from build123d import *

# Parameters (mm, degrees)
PAD003_DEPTH = 30
SKETCH005_R  = 6
POCKET_DEPTH = 30.001
SKETCH006_R  = 4.232151
PAD004_DEPTH = 20


with BuildPart() as part:
    # Sketch004 → Pad003 (new body)
    with BuildSketch(Plane.XY):
        Polygon((-12, 0), (-15, 0), (-15, 50), (15, 50), (15, 0), (12, 0), (12, 47), (-12, 47), align=None)
    extrude(amount=PAD003_DEPTH)

    # Sketch005 (on DatumPlane) → Pocket (cut, through all)
    with BuildSketch(Plane.YZ.offset(15)):
        with Locations((10, 15.016033)):
            Circle(SKETCH005_R)
    extrude(amount=-POCKET_DEPTH, mode=Mode.SUBTRACT)

    # Sketch006 (on DatumPlane) → Pad004 (join)
    with BuildSketch(Plane(origin=(0, 50, 0), x_dir=(-1, 0, 0), z_dir=(0, 1, 0))):
        with Locations((0, 15)):
            Circle(SKETCH006_R)
    extrude(amount=PAD004_DEPTH)


with BuildPart() as part_1:
    # Body009 placement: moved
    add(part.part.moved(Location((10, -300, 0))))


solid = part_1.part
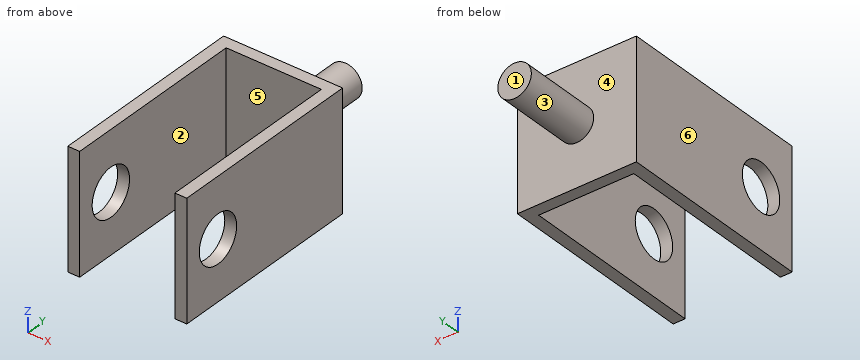
Source: CAD feature listing. Evaluate the final solid. Frame: model axes, mm. Face numbers are marked on the shaded views. A direction names the side the tool comes from. Coordinates: 2 decimals unless noted, no trailing zeros. Loops run counter-clockwise (first coordinate to the right, second up) from the corner with the lowest first, then second, coordinate; pieces in that order, holes last. Notation, with made-up numbers: (7, -33.5) - (11, -33.5) arc R22 cw to (11, -18.5) - close; hole circle Ø2 at (47.5, -13). An arc over 180 degrees is marked (long way). One line per question, with ' | ' between items.
1) Section C-C, the plane z = 22. Return loops of the section in (x, y).
Report:
outline: (-5, -300) - (-2, -300) - (-2, -253) - (22, -253) - (22, -300) - (25, -300) - (25, -250) - (-5, -250) - close
2) First-contact query: P1, Ø3, axis at x = 15.5, z = 4, coming from the -Y side; P2, Ø2, axis at y = -245.5, z = 21.5, coming from the +X side; P3, Ø3, axis at x = 14, z = 21.5, coming from the +Y side; P4, Ø15.5, axis at y = -290, z = 15.02, coming from the -X side. Flat tips, straight axial feed; report the tip coordinate or a pass-through.
Report:
P1: stops at y = -253 | P2: passes through | P3: stops at y = -250 | P4: stops at x = -5
3) Section A-A, the plane y = -280. Return loops of the section in (x, z), then the cut area to 3 significant figures.
Report:
outline: (-5, 0) - (-2, 0) - (-2, 30) - (-5, 30) - close; (22, 0) - (25, 0) - (25, 30) - (22, 30) - close | area: 180 mm²
4) Section B-B, the plane z = 10. Return loops of the section in (x, y), then the cut area to 3 significant figures.
Report:
outline: (-5, -300) - (-2, -300) - (-2, -293.29) - (-5, -293.29) - close; (-5, -286.71) - (-2, -286.71) - (-2, -253) - (22, -253) - (22, -286.71) - (25, -286.71) - (25, -250) - (-5, -250) - close; (22, -300) - (25, -300) - (25, -293.29) - (22, -293.29) - close | area: 332 mm²
5) Line query: line 1 along X through (y, z) = (-267.5, 18.5); line 2 along Z through (x, y) = (-3.2, -290); line 3 along Y through (x, z) = (18.5, 27.25). Output: solid intervals per line, ascending.
Report:
line 1: x = -5 to -2, 22 to 25 | line 2: z = 0 to 9.02, 21.02 to 30 | line 3: y = -253 to -250
6) Section D-D, the plane y = -290. Return loops of the section in (x, z).
Report:
outline: (-5, 0) - (-2, 0) - (-2, 9.02) - (-5, 9.02) - close; (-5, 21.02) - (-2, 21.02) - (-2, 30) - (-5, 30) - close; (22, 0) - (25, 0) - (25, 9.02) - (22, 9.02) - close; (22, 21.02) - (25, 21.02) - (25, 30) - (22, 30) - close
7) Set-up query: the marked faces 4, 5 and 6. Return all of +Z, -Z, +X, -X, +Y, -Y with unobstructed straight access to the full face (end or side cutting, diameter ignored); none if empty.
Report:
face 4: +Y | face 5: +Z, -Z, -Y | face 6: +Z, -Z, -X, +Y, -Y
8) Pull-direction query (X, two-part tool) for the marked faces 1, 2 and 3; classes: released by +X, released by -X, zero draft, split by the parting line, or undercut.
Report:
face 1: zero draft | face 2: undercut | face 3: split by the parting line
